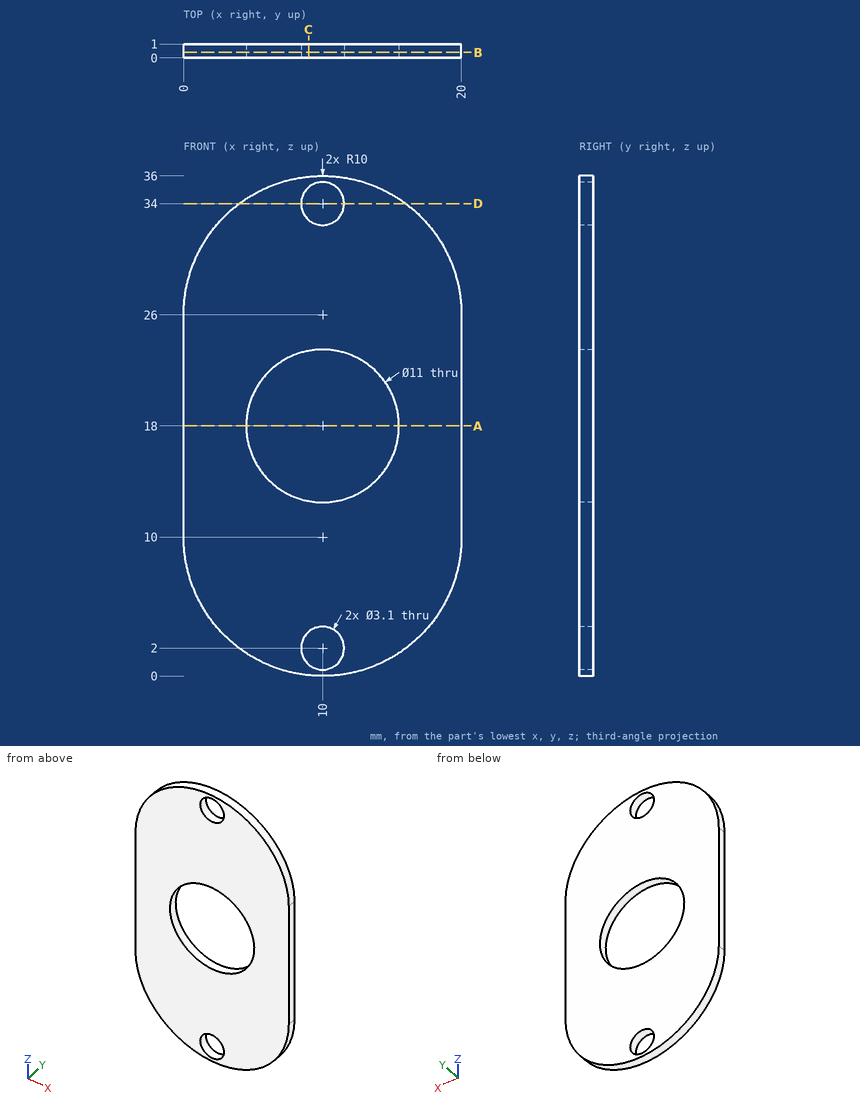
Geometry check sheet. Reference: drawing and pictorial views, mm from the part's lowest x, y, z. Coordinates: 2 decimals unless noted, no trailing zeros. Loops run counter-clockwise (first coordinate to the right, second up) from the corner with the lowest first, then second, coordinate; pieces in that order, holes last.
1) Gauge pin test, flat end, axial feed: pin 1 (3 mm diameter, centred on x = 10, z = 2, fed in from +Y). Record the tip position at first contact, or that the pin passes through.
2) Sectioned sample at A-A (z = 18). Record the boundary of the cut face in (x, y), and give its area (3 significant figures).
3) Sectioned sample at B-B (y = 0.4). Record the boundary of the cut face in (x, z), and give its area (3 significant figures).
4) Sectioned sample at C-C (x = 9). Record the boundary of the cut face in (y, z).
5) Sectioned sample at D-D (z = 34). Record the boundary of the cut face in (x, y).
6) Material ranges on probe 1 along Z at (x, y) = (10, 0.7); probe 2 along Z at (x, y) = (9, 0.7); probe 3 along X at (y, z) = (0.6, 18), recorded low to high.
Check sheet entries:
1. pin 1: passes through
2. outline: (0, 0) - (4.5, 0) - (4.5, 1) - (0, 1) - close; (15.5, 0) - (20, 0) - (20, 1) - (15.5, 1) - close
2. area: 9.00 mm2
3. outline: (0, 10) arc R10 ccw to (20, 10) - (20, 26) arc R10 ccw to (0, 26) - close; hole circle Ø11 at (10, 18); hole circle Ø3.1 at (10, 2); hole circle Ø3.1 at (10, 34)
3. area: 524 mm2
4. outline: (0, 0.05) - (1, 0.05) - (1, 0.82) - (0, 0.82) - close; (0, 3.18) - (1, 3.18) - (1, 12.59) - (0, 12.59) - close; (0, 23.41) - (1, 23.41) - (1, 32.82) - (0, 32.82) - close; (0, 35.18) - (1, 35.18) - (1, 35.95) - (0, 35.95) - close
5. outline: (4, 0) - (8.45, 0) - (8.45, 1) - (4, 1) - close; (11.55, 0) - (16, 0) - (16, 1) - (11.55, 1) - close
6. probe 1: z = 0 to 0.45, 3.55 to 12.5, 23.5 to 32.45, 35.55 to 36
6. probe 2: z = 0.05 to 0.82, 3.18 to 12.59, 23.41 to 32.82, 35.18 to 35.95
6. probe 3: x = 0 to 4.5, 15.5 to 20
